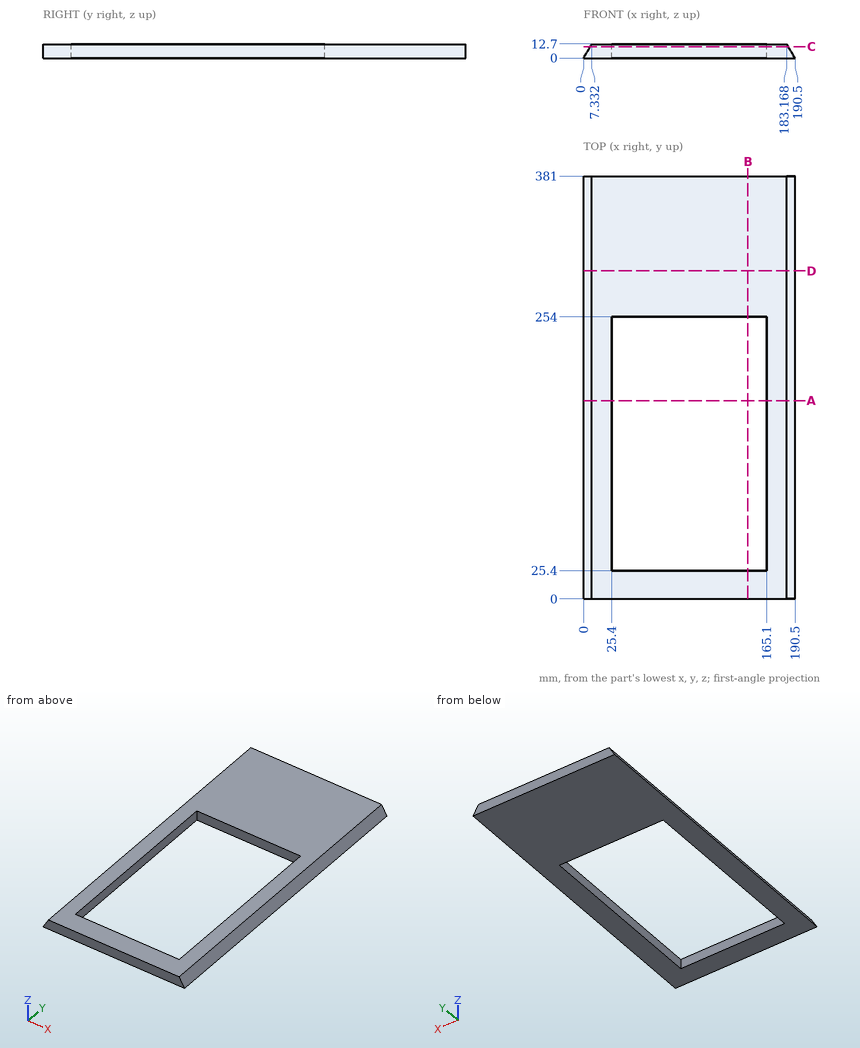
Geometry: see drawing. Coordinates: mm, zero at the bounding-box minimum. Coordinates: 2 decimals unless noted, no trailing zeros. Order: outer loops, then holes, each group sorted by start corner. A loop starts at its lowest first (then second) coordinate and runs counter-clockwise, first axis right, second up. Notation, with made-up numbers: M 22.5,87 L 35.5,87 A27 ccw 35.5,126 Z; hole C 55.5,61.5 d11. An arc over 180 degrees is marked long. Answer in a Markdown table with one row per item. Add a question column.
Q1. Section query A-A on y = 178.5. Return the cut outline in (x, z), and give its area (3 significant figures).
Q2. Line query: L1, parallel to Y at x = 60.5, z = 7.25; L2, parallel to X at y = 106.5, z = 9.25; L3, parallel to X at y = 200, z = 0.75. Output: solid intervals per line, ascending.
Q3. Section query D-D on y = 295.5. Return the cut outline in (x, z), and give its area (3 significant figures).
Q4. Contact query for flat-ended pins moving along their axis: P1, Ø3, axis at x = 142.5, z = 11, coming from the -Y side; P2, Ø6.5, axis at y = 128, z = 5.5, coming from the -X side; P3, Ø4, axis at y = 55, z = 10.5, coming from the -X side; P4, Ø4, axis at y = 196.5, z = 9.5, coming from the +X side. Output: stop coordinate, or through.
Q5. Section query C-C on z = 10.25. Return the cut outline in (x, y), and give its area (3 significant figures).
Q6. Section query B-B on x = 148. Return the cut outline in (y, z).
Completed:
| question | item | result |
|---|---|---|
| 1 | outline | M 0,0 L 25.4,0 L 25.4,12.7 L 7.33,12.7 Z; M 165.1,0 L 190.5,0 L 183.17,12.7 L 165.1,12.7 Z |
| 1 | area | 552 mm2 |
| 2 | L1 | y = 0 to 25.4, 254 to 381 |
| 2 | L2 | x = 5.34 to 25.4, 165.1 to 185.16 |
| 2 | L3 | x = 0.43 to 25.4, 165.1 to 190.07 |
| 3 | outline | M 0,0 L 190.5,0 L 183.17,12.7 L 7.33,12.7 Z |
| 3 | area | 2,330 mm2 |
| 4 | P1 | stops at y = 0 |
| 4 | P2 | stops at x = 1.3 |
| 4 | P3 | stops at x = 4.91 |
| 4 | P4 | stops at x = 186.17 |
| 5 | outline | M 5.92,0 L 184.58,0 L 184.58,381 L 5.92,381 Z; hole M 25.4,25.4 L 165.1,25.4 L 165.1,254 L 25.4,254 Z |
| 5 | area | 36,100 mm2 |
| 6 | outline | M 0,0 L 25.4,0 L 25.4,12.7 L 0,12.7 Z; M 254,0 L 381,0 L 381,12.7 L 254,12.7 Z |
